Read the model definition and answer for the solid it produces. Units are mm, in the model's axes. Coordinates: 2 decimals unless noted, no trailing zeros. Write each loop counter-clockwise with the first axis right and the second up, starting at its lowest first coordinate (ties: lowest second). Pieces come first, ordered by that corner, then holes. Notation, with made-up numbers: (2, 40) -> (42, 40) arc R17 ccw to (42, 59) -> close; hole circle Ø9 at (-19, -16.5). An arc over 180 degrees is marked (long way). Answer as a JSON object with one key per item and string values. Group by question number.
(1) Flat-ended cylindrical pins translate along their axes: P1, Ø0.8, axis at y = 1.5, z = 8, coming from the +X side; P2, Ø1, axis at x = 63, y = 1, coming from the +Z side. Find the tip coordinate at first contact, or state that the pin passes through.
(2) Find section C-C (z = -7). Give the vertices of the cut face in (x, y) (3 decimals).
(3) Straight lines are drawn through the part: L1, parallel to X at y = 2.9, z = -6; L2, parallel to Z at x = 60.25, y = 2.6; L3, parallel to Z at x = 60, y = 1.95. For each, find the intervals that lie inside material, in ascending order.
(4) Find section D-D (z = -21.5). Give the vertices of the cut face in (x, y) (3 decimals).
(5) Find section A-A (x = 64.25). Give the vertices of the cut face in (y, z) (3 decimals).
(6) Find section B-B (y = 2.3). Count the separate pieces of the cut face and the enclosed holes in it, then the cut area to 3 significant figures.
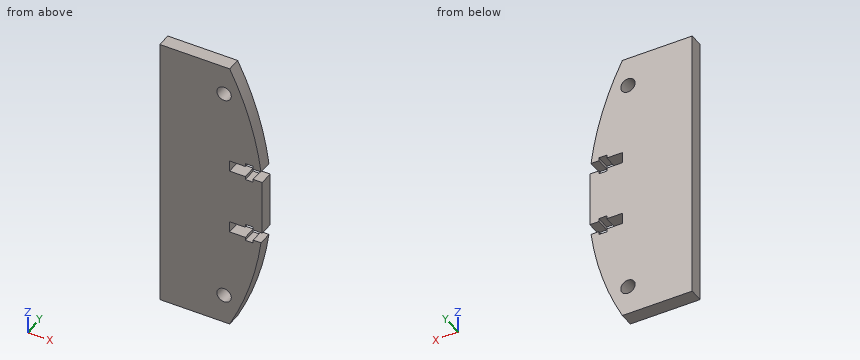
from build123d import *

# Parameters (mm, degrees)
SKETCH1_R           = 1.65
BOSS_EXTRUDE1_DEPTH = 3.175


with BuildPart() as part:
    # Sketch1 → Boss-Extrude1 (new body)
    with BuildSketch(Plane(origin=(0, 0, 0), x_dir=(1, 0, 0), z_dir=(0, 1, 0))):
        with BuildLine():
            Line((62.257529665, 32), (46.257529665, 32))
            Line((46.257529665, 32), (46.257529665, -32))
            Line((46.257529665, -32), (62.257529665, -32))
            ThreePointArc((62.257529665, -32), (66.851547843, -20.757421588), (69.43319019, -8.89))
            Line((69.43319019, -8.89), (67.63319019, -8.89))
            Line((67.63319019, -8.89), (67.63319019, -9.62))
            Line((67.63319019, -9.62), (65.83319019, -9.62))
            Line((65.83319019, -9.62), (65.83319019, -8.89))
            Line((65.83319019, -8.89), (62.23319019, -8.89))
            Line((62.23319019, -8.89), (62.23319019, -6.35))
            Line((62.23319019, -6.35), (65.83319019, -6.35))
            Line((65.83319019, -6.35), (65.83319019, -5.62))
            Line((65.83319019, -5.62), (67.63319019, -5.62))
            Line((67.63319019, -5.62), (67.63319019, -6.35))
            Line((67.63319019, -6.35), (69.711387162, -6.35))
            Line((69.711387162, -6.35), (69.711387162, 6.35))
            Line((69.711387162, 6.35), (67.63319019, 6.35))
            Line((67.63319019, 6.35), (67.63319019, 5.62))
            Line((67.63319019, 5.62), (65.83319019, 5.62))
            Line((65.83319019, 5.62), (65.83319019, 6.35))
            Line((65.83319019, 6.35), (62.23319019, 6.35))
            Line((62.23319019, 6.35), (62.23319019, 8.89))
            Line((62.23319019, 8.89), (65.83319019, 8.89))
            Line((65.83319019, 8.89), (65.83319019, 9.62))
            Line((65.83319019, 9.62), (67.63319019, 9.62))
            Line((67.63319019, 9.62), (67.63319019, 8.89))
            Line((67.63319019, 8.89), (69.43319019, 8.89))
            ThreePointArc((69.43319019, 8.89), (66.851547843, 20.757421588), (62.257529665, 32))
        make_face()
        with Locations((60.976049146, -25.257106536)):
            Circle(SKETCH1_R, mode=Mode.SUBTRACT)
        with Locations((60.976049146, 25.257106536)):
            Circle(SKETCH1_R, mode=Mode.SUBTRACT)
    extrude(amount=BOSS_EXTRUDE1_DEPTH)


solid = part.part
Results below:
{
 "1": {"P1": "stops at x = 62.23", "P2": "stops at z = 31.52"},
 "2": {"outline": "(46.258, 0) -> (62.233, 0) -> (62.233, 3.175) -> (46.258, 3.175) -> close"},
 "3": {"L1": "x = 46.26 to 65.83, 67.63 to 69.71", "L2": "z = -32 to -26.74, -23.78 to 23.78, 26.74 to 32", "L3": "z = -32 to -26.59, -23.93 to 23.93, 26.59 to 32"},
 "4": {"outline": "(46.258, 0) -> (66.616, 0) -> (66.616, 3.175) -> (46.258, 3.175) -> close"},
 "5": {"outline": "(0, -27.784) -> (3.175, -27.784) -> (3.175, -8.89) -> (0, -8.89) -> close; (0, -6.35) -> (3.175, -6.35) -> (3.175, 6.35) -> (0, 6.35) -> close; (0, 8.89) -> (3.175, 8.89) -> (3.175, 27.784) -> (0, 27.784) -> close"},
 "6": {"separate pieces": "1", "enclosed holes": "2", "area": "1,300 mm2"}
}
